```python
from build123d import *

# Parameters (mm, degrees)
F0_R     = 2.38125
F1_DEPTH = 7.9375
F3_DEPTH = 57.15
F4_R     = 19.05
F5_DEPTH = 9.525
F6_R     = 5.08


with BuildPart() as f1:
    # F0 (on Top) → F1 (new body)
    with BuildSketch(Plane.XY):
        with BuildLine():
            ThreePointArc((-18.0711051613, 33.4467460997), (-22.5612332218, 31.5868741602), (-24.4211051613, 27.0967460997))
            Line((-24.4211051613, 27.0967460997), (-24.4211051613, -17.3532539003))
            ThreePointArc((-24.4211051613, -17.3532539003), (-22.5612332218, -21.8433819608), (-18.0711051613, -23.7032539003))
            Line((-18.0711051613, -23.7032539003), (61.290320009, -23.7032539003))
            Line((61.290320009, -23.7032539003), (61.290320009, 33.4467460997))
            Line((61.290320009, 33.4467460997), (-18.0711051613, 33.4467460997))
        make_face()
        with Locations((-14.8961051613, -14.1782539003)):
            Circle(F0_R, mode=Mode.SUBTRACT)
        with Locations((-14.8961051613, 23.9217460997)):
            Circle(F0_R, mode=Mode.SUBTRACT)
    extrude(amount=-F1_DEPTH)

    # F2 (on face) → F3 (join)
    with BuildSketch(Plane.XZ.offset(23.7032539003)):
        Polygon((4.140320009, -7.9375), (-5.9959732738, -7.9375), (15.7223058273, -67.6079814199), (24.6728780403, -64.3502395547), align=None)
    extrude(amount=-F3_DEPTH)

    # F4 (on face) → F5 (cut, through all)
    with BuildSketch(Plane(origin=(-7.8456409666, 0, -2.8555797806), x_dir=(0, -1, 0), z_dir=(-0.9396926208, 0, -0.3420201433))):
        with Locations((-4.8717460997, -40.333066539)):
            Circle(F4_R)
        with BuildLine():
            ThreePointArc((-4.8717460546, -68.908066539), (-25.0773223561, -60.5386428273), (-33.4467460997, -40.333066539))
            Line((-33.4467460997, -40.333066539), (-33.4467460997, -68.908066539))
            Line((-33.4467460997, -68.908066539), (-4.8717460546, -68.908066539))
        make_face()
        with BuildLine():
            ThreePointArc((23.7032539003, -40.333066539), (15.3338301887, -60.5386427955), (-4.8717460546, -68.908066539))
            Line((-4.8717460546, -68.908066539), (23.7032539003, -68.908066539))
            Line((23.7032539003, -68.908066539), (23.7032539003, -40.333066539))
        make_face()
    extrude(amount=-F5_DEPTH, mode=Mode.SUBTRACT)

    # F6
    f6_edges = [f1.edges().sort_by_distance(p)[0] for p in [
        (-5.995973, 4.871746, -7.9375),
        (4.14032, 4.871746, -7.9375),
    ]]
    fillet(f6_edges, radius=F6_R)


solid = f1.part
```
Work out the finished part from the listing and answer in its coordinate system (mm). A direction names the side the tool comes from. Give positions to 0.01 mm unless a question says otherwise; leave off trailing zeros. Order: outer loops, then holes, each group sorted by start corner. A loop starts at its lowest first (then second) coordinate and runs counter-clockwise, first axis right, second up.
1. For faces 4 (the flat face through (16, -23.703, -5)), 5 (the flat face through (13.77, -14.58, -34.39)), determine the directions among +Z, -Z, +X, -X, +Y, -Y from which every point of the face is accessible in a straight line to the end or side of a thin tool.
Result sheet:
face 4: +Z, -Z, +X, -X, -Y
face 5: +X, +Y, -Y
2. Section C-C, the plane x = 47 is taken. Determine the outline of the cut face in (y, z).
Result sheet:
outline: (-23.7, -7.94) - (33.45, -7.94) - (33.45, 0) - (-23.7, 0) - close
3. The mould has two halves that part along Y. Classify faces 1 (the cylindrical face through (8.405, -13.299, -33.773)), 2 (the flat face through (-17, 5, -7.938)), 3 (the cylindrical face through (-22.51, 31.64, -3.91)): released by +Y, released by -Y, zero draft, split by the parting line, or undercut.
Result sheet:
face 1: undercut
face 2: zero draft
face 3: released by +Y
4. Straight lines are drawn through the part: L1, parallel to Z at x = 35, y = 16; L2, parallel to Y at x = 2.5, z = -29; L3, parallel to X at y = 19, z = -17. For each, find the intervals that lie inside material, in ascending order.
Result sheet:
L1: z = -7.94 to 0
L2: y = -23.7 to -9.74, 19.48 to 33.45
L3: x = -2.7 to 7.44
5. Section B-B, the plane y = 3.5 is taken. Determine the outline of the cut face in (x, z).
Result sheet:
outline: (-24.42, -7.94) - (-9.55, -7.94) arc R5.08 cw to (-4.78, -11.28) - (-0.55, -22.9) - (8.4, -19.64) - (6.62, -14.75) arc R5.08 cw to (11.4, -7.94) - (61.29, -7.94) - (61.29, 0) - (-24.42, 0) - close; (12.45, -58.61) - (15.71, -67.58) - (24.66, -64.32) - (21.4, -55.35) - close
6. Section A-A, the plane y = -10.5 is taken. Determine the outline of the cut face in (x, z), and give its area (3 significant figures).
Result sheet:
outline: (-24.42, -7.94) - (-9.55, -7.94) arc R5.08 cw to (-4.78, -11.28) - (2.1, -30.18) - (11.05, -26.92) - (6.62, -14.75) arc R5.08 cw to (11.4, -7.94) - (61.29, -7.94) - (61.29, 0) - (-24.42, 0) - close; (9.8, -51.33) - (14.19, -63.39) - (23.14, -60.13) - (18.75, -48.07) - close
area: 1,030 mm2
7. Section D-D, the plane x = 10 is taken. Give the number of separate pieces and of enclosed holes in the cut face, and give its area (3 significant figures).
Result sheet:
separate pieces: 3
enclosed holes: 0
area: 1,070 mm2
8. Each of these flat-tipped pins is pushed along its axis until it touches: P1, Ø25, axis at x = 45, y = 11.5, coming from the -Z side; P2, Ø1, axis at x = 10, y = 25.5, coming from the +Z side; P3, Ø3, axis at x = -14.9, y = -14.18, coming from the +Z side; P4, Ø1.5, axis at x = -9, y = 27.5, coming from the -Z side. Where does it stop, or does it pass through?
Result sheet:
P1: stops at z = -7.94
P2: stops at z = 0
P3: passes through
P4: stops at z = -8.11
